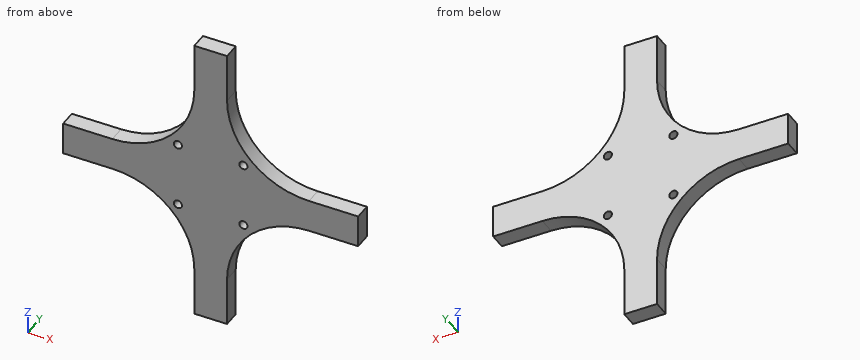
```python
from build123d import *

# Parameters (mm, degrees)
BOSS_EXTRUDE1_DEPTH = 25.4
CUT_EXTRUDE1_REACH  = 326.285
SKETCH2_R           = 6.35


with BuildPart() as part:
    # Sketch1 → Boss-Extrude1 (new body)
    with BuildSketch(Plane(origin=(0, 0, 0), x_dir=(1, 0, 0), z_dir=(0, 1, 0))):
        with BuildLine():
            Line((-152.4, 25.4), (-228.6, 25.4))
            Line((-228.6, 25.4), (-228.6, -25.4))
            Line((-228.6, -25.4), (-152.4, -25.4))
            ThreePointArc((-152.4, -25.4), (-62.597438789, -62.597438789), (-25.4, -152.4))
            Line((-25.4, -152.4), (-25.4, -228.6))
            Line((-25.4, -228.6), (25.4, -228.6))
            Line((25.4, -228.6), (25.4, -152.4))
            ThreePointArc((25.4, -152.4), (62.597438789, -62.597438789), (152.4, -25.4))
            Line((152.4, -25.4), (228.6, -25.4))
            Line((228.6, -25.4), (228.6, 25.4))
            Line((228.6, 25.4), (152.4, 25.4))
            ThreePointArc((152.4, 25.4), (62.597438789, 62.597438789), (25.4, 152.4))
            Line((25.4, 152.4), (25.4, 228.6))
            Line((25.4, 228.6), (-25.4, 228.6))
            Line((-25.4, 228.6), (-25.4, 152.4))
            ThreePointArc((-25.4, 152.4), (-62.597438789, 62.597438789), (-152.4, 25.4))
        make_face()
    extrude(amount=BOSS_EXTRUDE1_DEPTH)

    # Sketch2 → Cut-Extrude1 (cut, up to next)
    with BuildSketch(Plane(origin=(0, 0, 0), x_dir=(-1, 0, 0), z_dir=(0, -1, 0)), mode=Mode.PRIVATE) as cut_extrude1_sk1:
        with Locations(Location((50.8, -50.8, 0), (0, 0, 90))):
            Circle(SKETCH2_R)
    cut_extrude1_tool1 = extrude(cut_extrude1_sk1.sketch, amount=-CUT_EXTRUDE1_REACH, mode=Mode.PRIVATE) & part.part
    # Sketch2 → Cut-Extrude1 (cut, up to next)
    with BuildSketch(Plane(origin=(0, 0, 0), x_dir=(-1, 0, 0), z_dir=(0, -1, 0)), mode=Mode.PRIVATE) as cut_extrude1_sk2:
        with Locations(Location((50.8, 50.8, 0), (0, 0, 90))):
            Circle(SKETCH2_R)
    cut_extrude1_tool2 = extrude(cut_extrude1_sk2.sketch, amount=-CUT_EXTRUDE1_REACH, mode=Mode.PRIVATE) & part.part
    # Sketch2 → Cut-Extrude1 (cut, up to next)
    with BuildSketch(Plane(origin=(0, 0, 0), x_dir=(-1, 0, 0), z_dir=(0, -1, 0)), mode=Mode.PRIVATE) as cut_extrude1_sk3:
        with Locations(Location((-50.8, 50.8, 0), (0, 0, 90))):
            Circle(SKETCH2_R)
    cut_extrude1_tool3 = extrude(cut_extrude1_sk3.sketch, amount=-CUT_EXTRUDE1_REACH, mode=Mode.PRIVATE) & part.part
    # Sketch2 → Cut-Extrude1 (cut, up to next)
    with BuildSketch(Plane(origin=(0, 0, 0), x_dir=(-1, 0, 0), z_dir=(0, -1, 0)), mode=Mode.PRIVATE) as cut_extrude1_sk4:
        with Locations(Location((-50.8, -50.8, 0), (0, 0, 90))):
            Circle(SKETCH2_R)
    cut_extrude1_tool4 = extrude(cut_extrude1_sk4.sketch, amount=-CUT_EXTRUDE1_REACH, mode=Mode.PRIVATE) & part.part
    add(cut_extrude1_tool1.solids().sort_by_distance((-50.8, 0, 50.8))[0], mode=Mode.SUBTRACT)
    add(cut_extrude1_tool2.solids().sort_by_distance((-50.8, 0, -50.8))[0], mode=Mode.SUBTRACT)
    add(cut_extrude1_tool3.solids().sort_by_distance((50.8, 0, -50.8))[0], mode=Mode.SUBTRACT)
    add(cut_extrude1_tool4.solids().sort_by_distance((50.8, 0, 50.8))[0], mode=Mode.SUBTRACT)


solid = part.part
```
The listing builds one solid part. Answer for the finished solid, in the listing's coordinates (mm). Coordinates: 2 decimals unless noted, no trailing zeros. Loops run counter-clockwise (first coordinate to the right, second up) from the corner with the lowest first, then second, coordinate; pieces in that order, holes last. Notation, with made-up numbers: (73.25, -7.75) - (87.25, -7.75) arc R5 cw to (87.25, -2.75) - close; hole circle Ø1 at (30, 78.5). An arc over 180 degrees is marked (long way). Use a Markdown table: item, result. Add a question column.
1) The part is cut by section D-D, the plane z = 164.5. Give the vertices of the cut face in (x, y).
2) The part is cut by section C-C, the plane z = -50.8. Give the vertices of the cut face in (x, y).
3) The part is cut by section B-B, the plane y = 4.5. Give the vertices of the cut face in (x, z).
4) The part is cut by section A-A, the plane x = 50.8. Give the vertices of the cut face in (y, z), and give its area (3 significant figures).
5) Find the intervals of material crossed by line 1 (X direction, y = 17, z = 55); line 2 (X direction, y = 5.5, z = 50.8); line 3 (Z direction, x = 176, y = 6), in increasing order.
6) Given pin 1 (12 mm diameter, centred on y = 16, z = -170.5, fed in from -X); pin 2 (12.5 mm diameter, centred on x = 189.5, y = 12.5, fed in from -Z); pin 3 (3 mm diameter, centred on x = 70.5, y = 6, fed in from -Z); pin 4 (12 mm diameter, centred on x = -30, y = 22, fed in from +Z), each flat-ended and moving along its own axis, determine where each tip first touches the part or whether it passes through.
Here are the results:
| question | item | result |
|---|---|---|
| 1 | outline | (-25.4, 0) - (25.4, 0) - (25.4, 25.4) - (-25.4, 25.4) - close |
| 2 | outline | (-76.2, 0) - (-57.15, 0) - (-57.15, 25.4) - (-76.2, 25.4) - close; (-44.45, 0) - (44.45, 0) - (44.45, 25.4) - (-44.45, 25.4) - close; (57.15, 0) - (76.2, 0) - (76.2, 25.4) - (57.15, 25.4) - close |
| 3 | outline | (-228.6, -25.4) - (-152.4, -25.4) arc R127 cw to (-25.4, -152.4) - (-25.4, -228.6) - (25.4, -228.6) - (25.4, -152.4) arc R127 cw to (152.4, -25.4) - (228.6, -25.4) - (228.6, 25.4) - (152.4, 25.4) arc R127 cw to (25.4, 152.4) - (25.4, 228.6) - (-25.4, 228.6) - (-25.4, 152.4) arc R127 cw to (-152.4, 25.4) - (-228.6, 25.4) - close; hole circle Ø12.7 at (-50.8, -50.8); hole circle Ø12.7 at (-50.8, 50.8); hole circle Ø12.7 at (50.8, -50.8); hole circle Ø12.7 at (50.8, 50.8) |
| 4 | outline | (0, -76.2) - (25.4, -76.2) - (25.4, -57.15) - (0, -57.15) - close; (0, -44.45) - (25.4, -44.45) - (25.4, 44.45) - (0, 44.45) - close; (0, 57.15) - (25.4, 57.15) - (25.4, 76.2) - (0, 76.2) - close |
| 4 | area | 3,230 mm^2 |
| 5 | line 1 | x = -70.9 to -55.56, -46.04 to 46.04, 55.56 to 70.9 |
| 5 | line 2 | x = -76.2 to -57.15, -44.45 to 44.45, 57.15 to 76.2 |
| 5 | line 3 | z = -25.4 to 25.4 |
| 6 | pin 1 | stops at x = -25.4 |
| 6 | pin 2 | stops at z = -25.4 |
| 6 | pin 3 | stops at z = -56.62 |
| 6 | pin 4 | stops at z = 228.6 |
